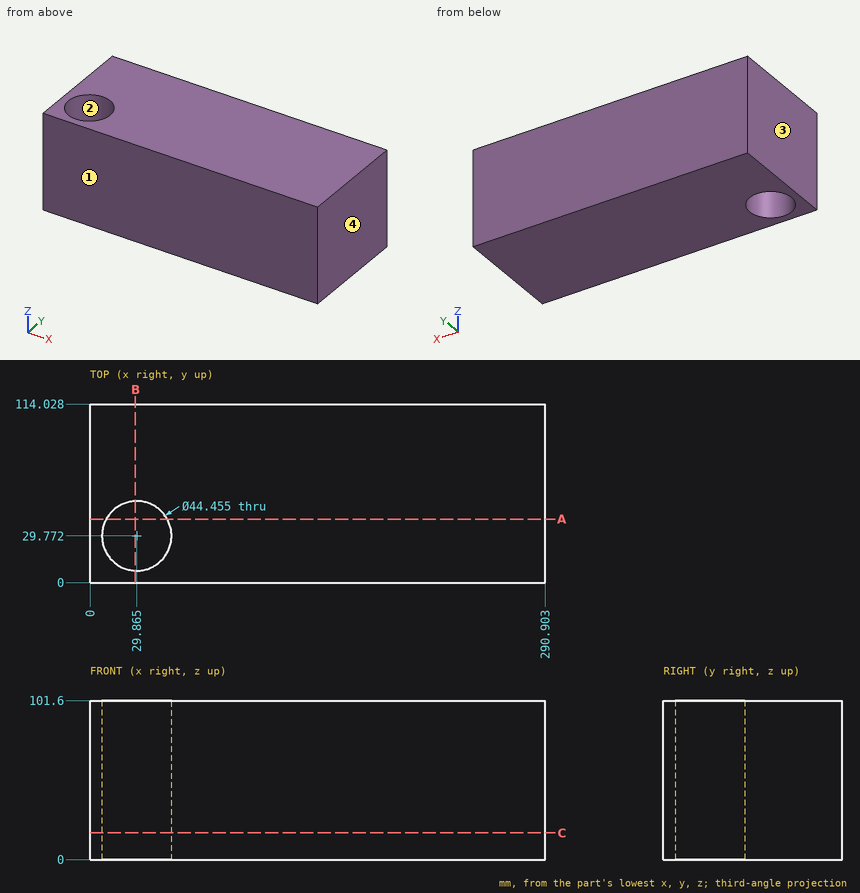
Print and shaded views of the part. All mm, measured from the part's lowest x, y and z. Coordinates: 2 decimals unless noted, no trailing zeros. Order: outer loops, then holes, each group sorted by start corner. A loop starts at its lowest first (then second) coordinate and runs counter-clockwise, first axis right, second up.
Item 1: Mould opens along X. For the marked faces 1, 2, 3 and 4 say: released by +X, released by -X, zero draft, split by the parting line, or undercut.
Filled in:
face 1: zero draft
face 2: undercut
face 3: released by -X
face 4: released by +X
Item 2: Drill centre lines: L1, parallel to X at y = 40, z = 9; L2, parallel to X at y = 31, z = 96.5; L3, parallel to Y at x = 13.5, z = 95.5 (1 decimal). Where is each one in solid material? Low to high.
Filled in:
L1: x = 0 to 10.13, 49.6 to 290.9
L2: x = 0 to 7.67, 52.06 to 290.9
L3: y = 0 to 14.7, 44.8 to 114
Item 3: Drop a flat-ended pin along its axis: pin 1 Ø12 at (x, y) = (173, 64) entering from -Z. Give the stop position or say it passes through.
Filled in:
pin 1: stops at z = 0
Item 4: Saw through at C-C on z = 17. List the corners of the cut face in (x, y) (1 decimal), then the cut area to 3 significant figures.
Filled in:
outline: (0, 0) - (290.9, 0) - (290.9, 114) - (0, 114) - close; hole circle Ø44.5 at (29.9, 29.8)
area: 31,600 mm2
Item 5: Saw through at B-B on x = 29. List the corners of the cut face in (y, z), then the cut area to 3 significant figures.
Filled in:
outline: (0, 0) - (7.56, 0) - (7.56, 101.6) - (0, 101.6) - close; (51.98, 0) - (114.03, 0) - (114.03, 101.6) - (51.98, 101.6) - close
area: 7,070 mm2
Item 6: Saw through at A-A on y = 40.5. List the corners of the cut face in (x, z), then the cut area to 3 significant figures.
Filled in:
outline: (0, 0) - (10.4, 0) - (10.4, 101.6) - (0, 101.6) - close; (49.33, 0) - (290.9, 0) - (290.9, 101.6) - (49.33, 101.6) - close
area: 25,600 mm2
